Geometry: final body of the model. Coordinates: model frame, mm. A direction names the side the tool comes from. Give positions to 0.01 mm unless a question says otherwise; leave off trailing zeros. Loops run counter-clockwise (first coordinate to the right, second up) from the corner with the lowest first, then second, coordinate; pieces in that order, holes last.
from build123d import *

# Parameters (mm, degrees)
SKETCH2_W           = 50
SKETCH2_H           = 41
BOSS_EXTRUDE1_DEPTH = 4
SKETCH4_W           = 152
SKETCH4_H           = 94
BOSS_EXTRUDE2_DEPTH = 14
CUT_EXTRUDE1_DEPTH  = 10
FILLET1_R           = 5
SKETCH5_W           = 4
SKETCH5_H           = 41
BOSS_EXTRUDE3_DEPTH = 80
CUT_EXTRUDE2_DEPTH  = 4
SKETCH7_R           = 2
CUT_EXTRUDE3_DEPTH  = 4
CHAMFER1_SIZE       = 1
FILLET2_R           = 5


with BuildPart() as part:
    # Sketch2 → Boss-Extrude1 (new body)
    with BuildSketch(Plane.XY):
        with Locations((25, 20.5)):
            Rectangle(SKETCH2_W, SKETCH2_H)
    extrude(amount=BOSS_EXTRUDE1_DEPTH)

    # Sketch4 → Boss-Extrude2 (add)
    with BuildSketch(Plane(origin=(0, 41, 0), x_dir=(1, 0, 0), z_dir=(0, 1, 0))):
        with Locations((25, -47)):
            Rectangle(SKETCH4_W, SKETCH4_H)
    extrude(amount=BOSS_EXTRUDE2_DEPTH)

    # 3DSketch1 → Cut-Extrude1 (cut)
    with BuildSketch(Plane(origin=(97, 55, 90), x_dir=(-0.8585432690668222, 0, -0.512741119026019), z_dir=(0, -1, 0))):
        Polygon((0, 0), (44.095736236, 73.83472114), (167.725966982, 0), (123.630230746, -73.83472114), align=None)
    extrude(amount=CUT_EXTRUDE1_DEPTH, mode=Mode.SUBTRACT)

    # Fillet1
    fillet1_edges = [part.edges().sort_by_distance(p)[0] for p in [
        (-51, 48, 94),
        (101, 48, 94),
    ]]
    fillet(fillet1_edges, radius=FILLET1_R)

    # Sketch5 → Boss-Extrude3 (add)
    with BuildSketch(Plane.XY.offset(4)):
        with Locations((25, 20.5)):
            Rectangle(SKETCH5_W, SKETCH5_H)
    extrude(amount=BOSS_EXTRUDE3_DEPTH)

    # Sketch6 → Cut-Extrude2 (cut)
    with BuildSketch(Plane(origin=(27, 0, 0), x_dir=(0, 0, -1), z_dir=(1, 0, 0))):
        Polygon((-4, 0), (-84, 0), (-84, 41), (-68, 41), (-4, 16), align=None)
    extrude(amount=-CUT_EXTRUDE2_DEPTH, mode=Mode.SUBTRACT)

    # Sketch7 → Cut-Extrude3 (cut)
    with BuildSketch(Plane.XY.offset(4)):
        with Locations((12.5, 8)):
            Circle(SKETCH7_R)
        with Locations((37.5, 8)):
            Circle(SKETCH7_R)
        with Locations(Location((37.5, 33, 0), (0, 0, 180))):
            Circle(SKETCH7_R)
        with Locations(Location((12.5, 33, 0), (0, 0, 180))):
            Circle(SKETCH7_R)
    extrude(amount=-CUT_EXTRUDE3_DEPTH, mode=Mode.SUBTRACT)

    # Chamfer1
    chamfer1_edges = [part.edges().sort_by_distance(p)[0] for p in [
        (10.5, 8, 4),
        (14.5, 33, 4),
        (39.5, 33, 4),
        (35.5, 8, 4),
    ]]
    chamfer(chamfer1_edges, length=CHAMFER1_SIZE)

    # Fillet2
    fillet2_edges = [part.edges().sort_by_distance(p)[0] for p in [
        (0, 41, 2),
        (50, 41, 2),
    ]]
    fillet(fillet2_edges, radius=FILLET2_R)


solid = part.part
Item 1: Section query B-B on z = 76. Return loops of the section in (x, y).
Values follow:
outline: (-51, 41) - (101, 41) - (101, 55) - (97, 55) - (97, 45) - (-47, 45) - (-47, 55) - (-51, 55) - close
Item 2: Section query D-D on y = 8. Return loops of the section in (x, z).
Values follow:
outline: (0, 0) - (10.5, 0) - (10.5, 3) - (9.5, 4) - (0, 4) - close; (14.5, 0) - (35.5, 0) - (35.5, 3) - (34.5, 4) - (15.5, 4) - (14.5, 3) - close; (39.5, 0) - (50, 0) - (50, 4) - (40.5, 4) - (39.5, 3) - close
Item 3: Section query C-C on x = 37.5. Return loops of the section in (y, z).
Values follow:
outline: (0, 0) - (6, 0) - (6, 3) - (5, 4) - (0, 4) - close; (10, 0) - (31, 0) - (31, 3) - (30, 4) - (11, 4) - (10, 3) - close; (35, 0) - (55, 0) - (55, 4) - (45, 4) - (45, 90) - (55, 90) - (55, 94) - (41, 94) - (41, 4) - (36, 4) - (35, 3) - close
Item 4: Draft query along Z for faces 5 (the face through (24, 48, 94)), 6 (the face through (7, 41, 46)), 7 (the face through (-47, 50, 46)). Return one class per face: +Z half, -Z half, draft (parallel to the pull), parting line (faces both ways), or undercut.
Values follow:
face 5: +Z half
face 6: draft
face 7: undercut
Item 5: Ray query, probe 1 along X at (y, z) = (33, 1.95); probe 2 along Y at (x, z) = (37.5, 1.2); probe 3 along Y at (x, z) = (37, 2). Return the intervals inside material, ascending.
Values follow:
probe 1: x = 0 to 10.5, 14.5 to 35.5, 39.5 to 50
probe 2: y = 0 to 6, 10 to 31, 35 to 55
probe 3: y = 0 to 6.06, 9.94 to 31.06, 34.94 to 55
Item 6: Pin query (flat end, axial travel): pin 1 (2.5 mm diameter, centred on x = 12.5, y = 33, fed in from +Z); pin 2 (20 mm diameter, centred on y = 23, z = 47.5, fed in from +X); pin 3 (4.5 mm diameter, centred on x = 12.5, y = 8, fed in from +Z); pin 4 (4.5 mm diameter, centred on y = 19.5, z = 1, fed in from +X). Return the tip coordinate at first contact, or that it passes through.
Values follow:
pin 1: passes through
pin 2: stops at x = 27
pin 3: stops at z = 3.25
pin 4: stops at x = 50
Item 7: Set-up query: faces 1 (the face through (27, 34, 21)), 2 (the face through (0, 18, 2)), 3 (the face through (50, 18, 2)), 4 (the face through (36.026, 9.352, 1.521)). Return all of +Z, -Z, +X, -X, +Y, -Y with unobstructed straight access to the full face (end or side cutting, diameter ignored); none if empty.
Values follow:
face 1: +Z, +X, -Y
face 2: +Z, -Z, -X, -Y
face 3: +Z, -Z, +X, -Y
face 4: +Z, -Z
Item 8: Section query A-A on y = 33. Return loops of the section in (x, z), plus the area to 3 significant figures.
Values follow:
outline: (0, 0) - (10.5, 0) - (10.5, 3) - (9.5, 4) - (0, 4) - close; (14.5, 0) - (35.5, 0) - (35.5, 3) - (34.5, 4) - (27, 4) - (27, 47.52) - (23, 47.52) - (23, 4) - (15.5, 4) - (14.5, 3) - close; (39.5, 0) - (50, 0) - (50, 4) - (40.5, 4) - (39.5, 3) - close
area: 340 mm2
